Work out the finished part from the listing and answer in its coordinate system (mm). A direction names the side the tool comes from. Give positions to 0.01 mm unless a question says otherwise; leave off trailing zeros. Loops run counter-clockwise (first coordinate to the right, second up) from the corner with the lowest first, then second, coordinate; pieces in that order, holes last. Notation, with made-up numbers: M 62,46.25 L 116,46.25 A22 cw 116,81.25 Z; hole C 28,84.25 d9. An arc over 180 degrees is marked long. Use a Markdown table: item, result.
```python
from build123d import *

# Parameters (mm, degrees)
BOSS_EXTRUDE1_DEPTH      = 15
CUT_EXTRUDE4_DEPTH       = 16
SKETCH8_R                = 2
CUT_EXTRUDE5_DEPTH       = 21.875
SKETCH9_W                = 8.175
SKETCH9_H                = 40
BOSS_EXTRUDE2_DEPTH      = 22.5
BOSS_EXTRUDE2_DEPTH_BACK = 7.5
SKETCH11_W               = 1.1
SKETCH11_H               = 20
CUT_EXTRUDE6_DEPTH       = 26
BOSS_EXTRUDE4_DEPTH      = 30
SKETCH13_W               = 1.9
SKETCH13_H               = 25
BOSS_EXTRUDE5_DEPTH      = 4
SKETCH15_W               = 5
SKETCH15_H               = 5
BOSS_EXTRUDE6_DEPTH      = 30
CUT_EXTRUDE7_DEPTH       = 23.5


with BuildPart() as part:
    # Sketch2 → Boss-Extrude1 (new body)
    with BuildSketch(Plane(origin=(0, 0, 0), x_dir=(0, 0, -1), z_dir=(1, 0, 0))):
        Polygon((0, 0), (0, 40), (-8.175, 40), (-8.175, 75), (-20.875, 75), (-20.875, 25), (-8.175, 25), (-8.175, 0), align=None)
    extrude(amount=BOSS_EXTRUDE1_DEPTH)

    # Sketch7 → Cut-Extrude4 (cut, through all)
    with BuildSketch(Plane.ZY):
        with BuildLine():
            Line((12.525, 75), (12.525, 63.615892333))
            ThreePointArc((12.525, 63.615892333), (14.525, 57.975), (16.525, 63.615892333))
            Line((16.525, 63.615892333), (16.525, 75))
            Line((16.525, 75), (12.525, 75))
        make_face()
    extrude(amount=-CUT_EXTRUDE4_DEPTH, mode=Mode.SUBTRACT)

    # Sketch8 → Cut-Extrude5 (cut, through all)
    with BuildSketch(Plane.XY.offset(20.875)):
        with Locations((7.5, 69)):
            Circle(SKETCH8_R)
    extrude(amount=-CUT_EXTRUDE5_DEPTH, mode=Mode.SUBTRACT)

    # Sketch9 → Boss-Extrude2 (add, two sides)
    with BuildSketch(Plane(origin=(0, 0, 0), x_dir=(0, 0, -1), z_dir=(1, 0, 0))) as boss_extrude2_sk:
        with Locations((-4.0875, 20)):
            Rectangle(SKETCH9_W, SKETCH9_H)
    extrude(amount=BOSS_EXTRUDE2_DEPTH)
    extrude(boss_extrude2_sk.sketch, amount=-BOSS_EXTRUDE2_DEPTH_BACK)

    # Sketch11 → Cut-Extrude6 (cut)
    with BuildSketch(Plane.ZY.offset(7.5)):
        with Locations((7.625, 12.5)):
            Rectangle(SKETCH11_W, SKETCH11_H)
    extrude(amount=-CUT_EXTRUDE6_DEPTH, mode=Mode.SUBTRACT)

    # Sketch12 → Boss-Extrude4 (add, through all)
    with BuildSketch(Plane.ZY.offset(7.5)):
        Polygon((10.075, 22.5), (7.075, 22.5), (7.075, 2.5), (10.075, 2.5), (10.075, 0), (5.075, 0), (5.075, 25), (10.075, 25), align=None)
    extrude(amount=-BOSS_EXTRUDE4_DEPTH)

    # Sketch13 → Boss-Extrude5 (add)
    with BuildSketch(Plane(origin=(22.5, 0, 0), x_dir=(0, 0, -1), z_dir=(1, 0, 0))):
        with Locations((-9.125, 12.5)):
            Rectangle(SKETCH13_W, SKETCH13_H)
    extrude(amount=-BOSS_EXTRUDE5_DEPTH)

    # Sketch15 → Boss-Extrude6 (add)
    with BuildSketch(Plane(origin=(22.5, 0, 0), x_dir=(0, 0, -1), z_dir=(1, 0, 0))):
        with Locations((-2.5, 11.65)):
            Rectangle(SKETCH15_W, SKETCH15_H)
    extrude(amount=BOSS_EXTRUDE6_DEPTH)

    # Sketch16 → Cut-Extrude7 (cut, through all)
    with BuildSketch(Plane(origin=(15, 0, 0), x_dir=(0, 0, -1), z_dir=(1, 0, 0))):
        Polygon((-10.075, 25), (-20.875, 43.706148722), (-20.875, 25), align=None)
    extrude(amount=-CUT_EXTRUDE7_DEPTH, mode=Mode.SUBTRACT)


solid = part.part
```
(1) A cutting plane is placed at A-A (y = 61.15). Write down the section's boundary in (x, z) (3 decimals), and give its area (4 significant figures).
Entries:
| item | result |
|---|---|
| outline | M 0,8.175 L 15,8.175 L 15,11.35 L 0,11.35 Z; M 0,17.7 L 15,17.7 L 15,20.875 L 0,20.875 Z |
| area | 95.25 mm² |
(2) The mould has two halves that part along Y. Classify faces 5 (the flat face through (5, 12, 7.075)), 6 (the flat face through (7, 75, 19)), 7 (the flat face through (19, 32, 8.175)), 8 (the flat face through (5, 2.5, 9)): released by +Y, released by -Y, zero draft, split by the parting line, or undercut.
Entries:
| item | result |
|---|---|
| face 5 | undercut |
| face 6 | released by +Y |
| face 7 | zero draft |
| face 8 | undercut |
(3) Consider probe 1 along Y at (x, z) = (8, 9); probe 2 along Z at (x, y) = (39, 13.5); probe 3 along Y at (x, z) = (7.5, 19.5). Determine where each line is inside the solid, lowest interval first. Write a range as [from, to].
Entries:
| item | result |
|---|---|
| probe 1 | y = [0, 2.5], [22.5, 67.06], [70.94, 75] |
| probe 2 | z = [0, 5] |
| probe 3 | y = [41.32, 67], [71, 75] |
(4) Which of the six approach directions +Z, -Z, +X, -X, +Y, -Y give full straight-line access (tool end or side, diameter ignored) to faces 1 (the flat face through (19, 11, 10.075)), 2 (the flat face through (37, 9.15, 3)), 3 (the flat face through (7, 57, 8.175)), 4 (the flat face through (37, 14.15, 3))?
Entries:
| item | result |
|---|---|
| face 1 | +Z, +X, -X, -Y |
| face 2 | +Z, -Z, +X, -Y |
| face 3 | -Z, +X, -X, +Y |
| face 4 | +Z, -Z, +X, +Y |
(5) A cutting plane is placed at C-C (y = 69). Write down the section's boundary in (x, z) (3 decimals).
Entries:
| item | result |
|---|---|
| outline | M 0,8.175 L 5.5,8.175 L 5.5,12.525 L 0,12.525 Z; M 0,16.525 L 5.5,16.525 L 5.5,20.875 L 0,20.875 Z; M 9.5,8.175 L 15,8.175 L 15,12.525 L 9.5,12.525 Z; M 9.5,16.525 L 15,16.525 L 15,20.875 L 9.5,20.875 Z |
(6) A cutting plane is placed at D-D (z = 2.75). Write down the section's boundary in (x, y).
Entries:
| item | result |
|---|---|
| outline | M -7.5,0 L 22.5,0 L 22.5,9.15 L 52.5,9.15 L 52.5,14.15 L 22.5,14.15 L 22.5,40 L -7.5,40 Z |
(7) Given P1, Ø1, axis at x = -1, z = 11.5, coming from the -Y side; P2, Ø4, axis at y = 44.5, z = 14, coming from the +X side; P3, Ø8, axis at x = -5, y = 30.5, coming from the +Z side (3 decimals); P4, Ø1.5, axis at x = 20, z = 9, coming from the +Y side, each flat-ended and moving along its own axis, determine where each tip first touches the part or whether it passes through.
Entries:
| item | result |
|---|---|
| P1 | passes through |
| P2 | stops at x = 15 |
| P3 | stops at z = 8.175 |
| P4 | stops at y = 25 |
(8) A cutting plane is placed at B-B (x = 7.5). Write down the section's boundary in (y, z) (3 decimals).
Entries:
| item | result |
|---|---|
| outline | M 0,0 L 40,0 L 40,8.175 L 67,8.175 L 67,12.525 L 63.616,12.525 A3.175 cw long 63.616,16.525 L 67,16.525 L 67,20.875 L 43.706,20.875 L 25,10.075 L 22.5,10.075 L 22.5,7.075 L 2.5,7.075 L 2.5,10.075 L 0,10.075 Z; M 71,8.175 L 75,8.175 L 75,12.525 L 71,12.525 Z; M 71,16.525 L 75,16.525 L 75,20.875 L 71,20.875 Z |
